```python
from build123d import *

# Parameters (mm, degrees)
F0_W           = 25
F0_H           = 25
F1_DEPTH       = 15
F2_SIZE        = 4
F4_D           = 5.2
F4_CBORE_D     = 9.75
F4_CBORE_DEPTH = 8


with BuildPart() as f1:
    # F0 (on Top) → F1 (new body)
    with BuildSketch(Plane.XY):
        Rectangle(F0_W, F0_H)
    extrude(amount=F1_DEPTH)

    # F2
    f2_edges = [f1.edges().sort_by_distance(p)[0] for p in [
        (-12.5, 0, 15),
        (0, 12.5, 15),
        (12.5, 0, 15),
        (0, -12.5, 15),
    ]]
    chamfer(f2_edges, length=F2_SIZE)

    # F4 (through all)
    with Locations(Plane.XY.offset(15)):
        with Locations((0, 0)):
            CounterBoreHole(F4_D / 2, F4_CBORE_D / 2, F4_CBORE_DEPTH)


solid = f1.part
```
Verification items for the finished model (mm, model axes). A direction names the side the tool comes from. Round coordinates to 2 decimals unless told otherwise and drop trailing zeros. Write each loop counter-clockwise with the first axis right and the second up, starting at its lowest first coordinate (ties: lowest second). Pieces come first, ordered by that corner, then holes. Notation, with made-up numbers: (45.5, 30.25) - (78.5, 30.25) arc R26 cw to (78.5, 47.25) - close; hole circle Ø4 at (65.5, 45). An arc over 180 degrees is marked (long way). Answer as a JSON object with one key per item and string values. Group by question number.
Q1. Thickness scan on line 1 (Y direction, x = 0, z = 10) (3 decimals); line 2 (X direction, y = 0.25, z = 11); line 3 (Z direction, x = -3, y = 2.5). Record the ranges inside material, lowest first.
Q2. Mould release check, pull along X, two halves, no side actions. Record for faces 3 (the cylindrical face through (0.338, 2.578, 3.451)), 4 (the cylindrical face through (-0.635, 4.834, 11.056)), 5 (the flat face through (0, -12.5, 5)), 6 (the flat face through (-10.5, -0.2, 13)): released by +X, released by -X, zero draft, split by the parting line, or undercut.
Q3. Tool access check on faces 1 (the flat face through (2, -2, 7)), 2 (the flat face through (-12.5, 0, 5)). Record the directions out of +Z, -Z, +X, -X, +Y, -Y that give a thin tool (end or side, any length) a straight path to the whole face; none if there is none.
Q4. Section check D-D, the plane x = -9.75. Enter the section's corners in (y, z), plus the area to 3 significant figures.
Q5. Section check A-A, the plane x = 0. Enter the section's corners in (y, z) (3 decimals).
Q6. Section check C-C, the plane z = 5.5. Enter the section's corners in (x, y).
Q7. Section check B-B, the plane y = 1.75. Enter the section's corners in (x, z), plus the area to 3 significant figures.
Q8. Go/stop test with flat-tipped pins: pin 1 Ø10 at (x, y) = (-6.5, 0) entering from -Z; pin 2 Ø5 at (x, y) = (0, -0.5) entering from +Z. Record where each tip stops, or that it passes through.
Found:
{
 "1": {"line 1": "y = -12.5 to -4.875, 4.875 to 12.5", "line 2": "x = -12.5 to -4.87, 4.87 to 12.5", "line 3": "z = 0 to 7"},
 "2": {"face 3": "undercut", "face 4": "undercut", "face 5": "zero draft", "face 6": "released by -X"},
 "3": {"face 1": "+Z", "face 2": "+Z, -Z, -X, +Y, -Y"},
 "4": {"outline": "(-12.5, 0) - (12.5, 0) - (12.5, 11) - (9.75, 13.75) - (-9.75, 13.75) - (-12.5, 11) - close", "area": "336 mm^2"},
 "5": {"outline": "(-12.5, 0) - (-2.6, 0) - (-2.6, 7) - (-4.875, 7) - (-4.875, 15) - (-8.5, 15) - (-12.5, 11) - close; (2.6, 0) - (12.5, 0) - (12.5, 11) - (8.5, 15) - (4.875, 15) - (4.875, 7) - (2.6, 7) - close"},
 "6": {"outline": "(-12.5, -12.5) - (12.5, -12.5) - (12.5, 12.5) - (-12.5, 12.5) - close; hole circle Ø5.2 at (0, 0)"},
 "7": {"outline": "(-12.5, 0) - (-1.92, 0) - (-1.92, 7) - (-4.55, 7) - (-4.55, 15) - (-8.5, 15) - (-12.5, 11) - close; (1.92, 0) - (12.5, 0) - (12.5, 11) - (8.5, 15) - (4.55, 15) - (4.55, 7) - (1.92, 7) - close", "area": "259 mm^2"},
 "8": {"pin 1": "stops at z = 0", "pin 2": "stops at z = 7"}
}
